```python
from build123d import *

# Parameters (mm, degrees)
SKETCH1_W           = 40
SKETCH1_H           = 14
BOSS_EXTRUDE1_DEPTH = 40
CUT_EXTRUDE1_DEPTH  = 74


with BuildPart() as part:
    # Sketch1 → Boss-Extrude1 (new, symmetric)
    with BuildSketch(Plane(origin=(0, 0, 0), x_dir=(1, 0, 0), z_dir=(0, 1, 0))):
        Rectangle(SKETCH1_W, SKETCH1_H)
    extrude(amount=BOSS_EXTRUDE1_DEPTH, both=True)

    # Sketch3 → Cut-Extrude1 (cut)
    with BuildSketch(Plane(origin=(0, 34, 0), x_dir=(1, 0, 0), z_dir=(0, 1, 0))):
        Polygon((-16.025, 1.05), (16.025, 1.05), (11.923320132, -7), (-11.923320132, -7), align=None)
    extrude(amount=-CUT_EXTRUDE1_DEPTH, mode=Mode.SUBTRACT)


solid = part.part
```
Model file for the job. Use its own axes, mm. A direction names the side the tool comes from. Coordinates: 2 decimals unless noted, no trailing zeros. Order: outer loops, then holes, each group sorted by start corner. A loop starts at its lowest first (then second) coordinate and runs counter-clockwise, first axis right, second up. Notation, with made-up numbers: (17.25, 74.5) -> (67.25, 74.5) arc R14 cw to (67.25, 86.5) -> close; hole circle Ø2 at (80.25, -11). An arc over 180 degrees is marked (long way). Answer as a JSON object with one key per item and string values. Group by question number.
1) Cut at B-B, the plane x = 3. Write the cut outline in (y, z), then the cut area to 3 significant figures.
2) Pull direction X, two halves, no side cores. Call faces 3 (the face through (0, 40, 0)), 4 (the face through (20, 1, 0)), 5 (the face through (14, -2.48, 2.92)): +X half, -X half, draft (parallel to the pull), parting line (faces both ways), or undercut.
3) Flat gauge pins, fed straight in: pin 1 (2 mm diameter, centred on x = -11, z = 1.5, fed in from -Y); pin 2 (2 mm diameter, centred on x = 3.5, y = 14, fed in from +Z). Where does each tip first touch, or does it go through?
4) Cut at C-C, the plane z = 0.25. Write the cut outline in (x, y).
5) Cut at A-A, the plane y = 29.5. Write the cut outline in (x, z) (3 decimals).
6) Which spindle directions (+Z, -Z, +X, -X, +Y, -Y) get a long thin tool onto all of the face, cutting with end or side? Do faces 1 (the face through (0, 1, -7)), 2 (the face through (-13.945, -2.482, 3.031)). Say none if no direction does.
7) Drill centre lines: L1, parallel to Z at x = 14, y = 11.5; L2, parallel to Z at x = 2, y = -27; L3, parallel to Z at x = -15, y = -11. Where is each one in solid material? Low to high.
Check values:
{
 "1": {"outline": "(-40, -7) -> (40, -7) -> (40, 7) -> (34, 7) -> (34, -1.05) -> (-40, -1.05) -> close", "area": "524 mm²"},
 "2": {"face 3": "draft", "face 4": "+X half", "face 5": "undercut"},
 "3": {"pin 1": "stops at y = 34", "pin 2": "stops at z = -1.05"},
 "4": {"outline": "(-20, -40) -> (-15.36, -40) -> (-15.36, 34) -> (15.36, 34) -> (15.36, -40) -> (20, -40) -> (20, 40) -> (-20, 40) -> close"},
 "5": {"outline": "(-20, -7) -> (20, -7) -> (20, 7) -> (11.923, 7) -> (16.025, -1.05) -> (-16.025, -1.05) -> (-11.923, 7) -> (-20, 7) -> close"},
 "6": {"face 1": "-Z, +X, -X, +Y, -Y", "face 2": "-Y"},
 "7": {"L1": "z = -7 to -1.05, 2.92 to 7", "L2": "z = -7 to -1.05", "L3": "z = -7 to -1.05, 0.96 to 7"}
}
